Source: CAD feature listing. Evaluate the final solid. Frame: model axes, mm. A direction names the side the tool comes from. Round coordinates to 2 decimals unless told otherwise and drop trailing zeros. Write each loop counter-clockwise with the first axis right and the second up, starting at its lowest first coordinate (ties: lowest second). Pieces come first, ordered by that corner, then holes. Notation, with made-up numbers: M 51.5,19 L 106.5,19 A27 cw 106.5,36 Z; hole C -24.5,60.5 d3. An arc over 180 degrees is marked long. Answer in a Markdown table with one row per item.
from build123d import *

# Parameters (mm, degrees)
PAD_DEPTH       = 6
SKETCH001_W     = 12.5
SKETCH001_H     = 23
POCKET_DEPTH    = 12.001
SKETCH002_W     = 13
SKETCH002_H     = 39
POCKET001_DEPTH = 4


with BuildPart() as part:
    # Sketch → Pad (new body, symmetric)
    with BuildSketch(Plane.XZ):
        with BuildLine():
            Line((-14, 0), (-14, 2))
            Line((-14, 2), (-8.5, 2))
            Line((-8.5, 2), (-8.5, 36.5))
            ThreePointArc((8.5, 36.5), (0, 39.380883), (-8.5, 36.5))
            Line((8.5, 2), (8.5, 36.5))
            Line((8.5, 2), (14, 2))
            Line((14, 2), (14, 0))
            Line((14, 0), (-14, 0))
        make_face()
    extrude(amount=PAD_DEPTH, both=True)

    # Sketch001 (on Face10 of Pad) → Pocket (cut, through all)
    with BuildSketch(Plane.XZ.offset(6)):
        with Locations((0, 18.3)):
            Rectangle(SKETCH001_W, SKETCH001_H)
    extrude(amount=-POCKET_DEPTH, mode=Mode.SUBTRACT)

    # Sketch002 (on Face5 of Pocket) → Pocket001 (cut)
    with BuildSketch(Plane.XZ.offset(6)):
        with Locations((0, 21.5)):
            Rectangle(SKETCH002_W, SKETCH002_H)
    pocket001 = extrude(amount=-POCKET001_DEPTH, mode=Mode.SUBTRACT)

    # Mirrored: Pocket001 across XZ
    add(pocket001.mirror(Plane.XZ), mode=Mode.SUBTRACT)


solid = part.part
Q1. Section D-D (y = -5). Return loops of the section in (x, z).
Solutions:
| item | result |
|---|---|
| outline | M -14,0 L 14,0 L 14,2 L 8.5,2 L 8.5,36.5 A13.98 ccw 6.5,37.78 L 6.5,2 L -6.5,2 L -6.5,37.78 A13.98 ccw -8.5,36.5 L -8.5,2 L -14,2 Z |
Q2. Material intervals for probe 1 along X at (y, z) = (5.75, 24); probe 2 along X at (y, z) = (0.25, 29.5); probe 3 along Y at (x, z) = (-3.25, 3), sorted ascending.
Solutions:
| item | result |
|---|---|
| probe 1 | x = -8.5 to -6.5, 6.5 to 8.5 |
| probe 2 | x = -8.5 to -6.25, 6.25 to 8.5 |
| probe 3 | y = -2 to 2 |
Q3. Pull-direction query (Z, two-part tool) for faces 5 (the flat face through (0, 0, 29.8)), 6 (the flat face through (8.5, 0, 19)), 7 (the flat face through (-11, 0, 2)); classes: pulls with the +Z half, pulls with the -Z half, needs draft (parallel to the pull), parting line crosses it, or undercut.
Solutions:
| item | result |
|---|---|
| face 5 | undercut |
| face 6 | needs draft |
| face 7 | pulls with the +Z half |
Q4. Section A-A (z = 12.5). Return loops of the section in (x, y), and give its area (3 significant figures).
Solutions:
| item | result |
|---|---|
| outline | M -8.5,-6 L -6.5,-6 L -6.5,-2 L -6.25,-2 L -6.25,2 L -6.5,2 L -6.5,6 L -8.5,6 Z; M 6.25,-2 L 6.5,-2 L 6.5,-6 L 8.5,-6 L 8.5,6 L 6.5,6 L 6.5,2 L 6.25,2 Z |
| area | 50.0 mm2 |
Q5. Section C-C (y = -0.75). Return loops of the section in (x, z).
Solutions:
| item | result |
|---|---|
| outline | M -14,0 L 14,0 L 14,2 L 8.5,2 L 8.5,36.5 A13.98 ccw -8.5,36.5 L -8.5,2 L -14,2 Z; hole M -6.25,6.8 L 6.25,6.8 L 6.25,29.8 L -6.25,29.8 Z |
Q6. Section B-B (x = -2.5). Return loops of the section in (y, z), and give its area (3 significant figures).
Solutions:
| item | result |
|---|---|
| outline | M -6,0 L 6,0 L 6,2 L 2,2 L 2,6.8 L -2,6.8 L -2,2 L -6,2 Z; M -2,29.8 L 2,29.8 L 2,39.16 L -2,39.16 Z |
| area | 80.6 mm2 |
Q7. Contact query for flat-ended pins moving along their axis: pin 1 Ø3 at (x, y) = (-1.5, 0.5) entering from +Z; pin 2 Ø3 at (x, y) = (11, -3) entering from +Z; pin 3 Ø1.2 at (y, z) = (3.5, 12.5) entering from +X; pin 4 Ø2 at (y, z) = (5, 13.5) entering from -X. Output: stop coordinate, or through.
Solutions:
| item | result |
|---|---|
| pin 1 | stops at z = 39.38 |
| pin 2 | stops at z = 2 |
| pin 3 | stops at x = 8.5 |
| pin 4 | stops at x = -8.5 |
Q8. Access query for faces 1 (the flat face through (-6.5, 4, 20)), 2 (the flat face through (11, 0, 2)), 3 (the flat face through (-6.25, 0, 18)), 4 (the flat face through (-8.5, 0, 19)). Directions: +Z, -Z, +X, -X, +Y, -Y. A direction counts if a zero-diameter tool reaches every point of the face in a straight line with its end or side. Return the directions, or none.
Solutions:
| item | result |
|---|---|
| face 1 | +Z, +Y |
| face 2 | +Z, +X, +Y, -Y |
| face 3 | +Y, -Y |
| face 4 | +Z, -X, +Y, -Y |
